The figure shows three views and two pictorial views of one solid part (mm, origin at its lowest corner). Answer the questions. Coordinates: 2 decimals unless noted, no trailing zeros. Loops run counter-clockwise (first coordinate to the right, second up) from the corner with the lowest first, then second, coordinate; pieces in that order, holes last. Notation, with made-up numbers: M -36,44 L 18,44 A17 ccw 18,48 Z; hole C 1.25,38.5 d1. An arc over 180 degrees is marked long. Answer in a Markdown table with one row per item. Add a question column.
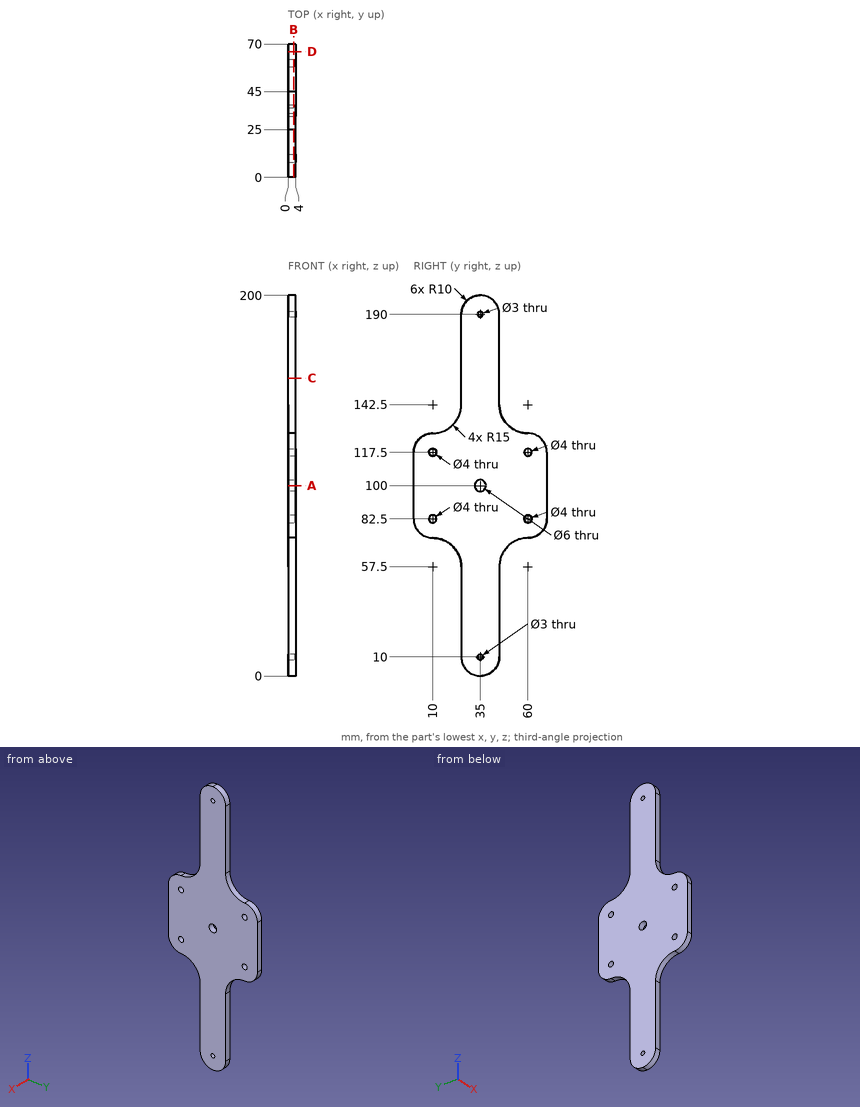
(1) A cutting plane is placed at D-D (y = 66). Give the vertices of the cut face in (x, z), plus the area to 3 significant figures.
(2) Each of these flat-tipped pins is pushed along its axis until it touches: pin 1 (1 mm diameter, centred on x = 1, y = 54, fed in from -Z); pin 2 (2 mm diameter, centred on x = 2.5, z = 30, fed in from +Y); pin 3 (1.5 mm diameter, centred on x = 1, y = 26, fed in from +Z). Where does it stop, or does it pass through?
(3) A cutting plane is placed at C-C (z = 156.5). Give the vertices of the cut face in (x, y).
(4) A cutting plane is placed at A-A (z = 100). Give the vertices of the cut face in (x, y), plus the area to 3 significant figures.
(5) Straight lines are drawn through the part: line 1 (Z direction, x = 1.75, y = 10); line 2 (Y direction, x = 3.6, z = 144); line 3 (Y direction, x = 2.45, z = 190). For each, find the intervals that lie inside material, in ascending order.
(6) A cutting plane is placed at B-B (x = 2.95). Give the vertices of the cut face in (y, z).
Solved:
| question | item | result |
|---|---|---|
| 1 | outline | M 0,74.5 L 4,74.5 L 4,125.5 L 0,125.5 Z |
| 1 | area | 204 mm² |
| 2 | pin 1 | stops at z = 71.02 |
| 2 | pin 2 | stops at y = 45 |
| 2 | pin 3 | stops at z = 195.65 |
| 3 | outline | M 0,25 L 4,25 L 4,45 L 0,45 Z |
| 4 | outline | M 0,0 L 4,0 L 4,32 L 0,32 Z; M 0,38 L 4,38 L 4,70 L 0,70 Z |
| 4 | area | 256 mm² |
| 5 | line 1 | z = 72.5 to 80.5, 84.5 to 115.5, 119.5 to 127.5 |
| 5 | line 2 | y = 25 to 45 |
| 5 | line 3 | y = 25 to 33.5, 36.5 to 45 |
| 6 | outline | M 0,82.5 A10 ccw 10,72.5 A15 cw 25,57.5 L 25,10 A10 ccw 45,10 L 45,57.5 A15 cw 60,72.5 A10 ccw 70,82.5 L 70,117.5 A10 ccw 60,127.5 A15 cw 45,142.5 L 45,190 A10 ccw 25,190 L 25,142.5 A15 cw 10,127.5 A10 ccw 0,117.5 Z; hole C 10,82.5 d4; hole C 10,117.5 d4; hole C 35,100 d6; hole C 35,10 d3; hole C 35,190 d3; hole C 60,82.5 d4; hole C 60,117.5 d4 |
